```python
from build123d import *

# Parameters (mm, degrees)
SKETCH2_R           = 11.5
BOSS_EXTRUDE1_DEPTH = 1
SKETCH3_R           = 10
BOSS_EXTRUDE2_DEPTH = 4
SKETCH4_R           = 2.525
CUT_EXTRUDE1_DEPTH  = 17.984370982
SKETCH5_R           = 2
CUT_EXTRUDE2_DEPTH  = 0.3
CIRPATTERN1_COUNT   = 14
SKETCH7_R           = 10
SKETCH7_R_2         = 2.525
BOSS_EXTRUDE4_DEPTH = 1.5
BOSS_EXTRUDE3_DEPTH = 0.998
SKETCH8_R           = 1.1
CUT_EXTRUDE3_DEPTH  = 2.69
CUT_EXTRUDE4_DEPTH  = 1.7
CIRPATTERN2_COUNT   = 3
SKETCH11_R          = 11.5
BOSS_EXTRUDE5_DEPTH = 3
SKETCH12_R          = 1.65
CUT_EXTRUDE5_DEPTH  = 4
CUT_EXTRUDE6_DEPTH  = 2.8
CIRPATTERN3_COUNT   = 4
SKETCH16_R          = 4.5
CUT_EXTRUDE9_DEPTH  = 2
SKETCH17_R          = 3.5
CUT_EXTRUDE10_DEPTH = 18.866109191


with BuildPart() as part:
    # Sketch2 → Boss-Extrude1 (new body)
    with BuildSketch(Plane(origin=(0, 0, 0), x_dir=(1, 0, 0), z_dir=(0, 1, 0))):
        with Locations(Location((0, 0, 0), (0, 0, 270))):
            Circle(SKETCH2_R)
    extrude(amount=BOSS_EXTRUDE1_DEPTH)

    # Sketch3 → Boss-Extrude2 (add)
    with BuildSketch(Plane(origin=(0, 1, 0), x_dir=(1, 0, 0), z_dir=(0, 1, 0))):
        with Locations(Location((0, 0, 0), (0, 0, 270))):
            Circle(SKETCH3_R)
    extrude(amount=BOSS_EXTRUDE2_DEPTH)

    # Sketch4 → Cut-Extrude1 (cut, through all)
    with BuildSketch(Plane(origin=(0, 4.8958, 0), x_dir=(-1, 0, 0), z_dir=(0, -1, 0))):
        with Locations(Location((0, 7, 0), (0, 0, 90))):
            Circle(SKETCH4_R)
    cut_extrude1 = extrude(amount=-CUT_EXTRUDE1_DEPTH, mode=Mode.SUBTRACT)

    # Sketch5 → Cut-Extrude2 (cut)
    with BuildSketch(Plane(origin=(0, 4.8958, 0), x_dir=(1, 0, 0), z_dir=(0, 1, 0))):
        with Locations(Location((0, 7, 0), (0, 0, 270))):
            Circle(SKETCH5_R)
    cut_extrude2 = extrude(amount=-CUT_EXTRUDE2_DEPTH, mode=Mode.SUBTRACT)

    # CirPattern1: Cut-Extrude1, Cut-Extrude2 ×14 about axis, 11 skipped
    cirpattern1_axis = Axis((0, 5, 0), (0, -1, 0))
    add([cut_extrude1.rotate(cirpattern1_axis, i * 360 / CIRPATTERN1_COUNT) for i in range(1, CIRPATTERN1_COUNT) if i not in (1, 2, 3, 4, 6, 7, 8, 10, 11, 12, 13)], mode=Mode.SUBTRACT)
    add([cut_extrude2.rotate(cirpattern1_axis, i * 360 / CIRPATTERN1_COUNT) for i in range(1, CIRPATTERN1_COUNT) if i not in (1, 2, 3, 4, 6, 7, 8, 10, 11, 12, 13)], mode=Mode.SUBTRACT)

    # Sketch7 → Boss-Extrude4 (add)
    with BuildSketch(Plane(origin=(0, 4.8958, 0), x_dir=(1, 0, 0), z_dir=(0, 1, 0))):
        with Locations(Location((0, 0, 0), (0, 0, 270))):
            Circle(SKETCH7_R)
        with Locations(Location((5.472820377, -4.364428613, 0), (0, 0, 321.428571429))):
            Circle(SKETCH7_R_2, mode=Mode.SUBTRACT)
        with Locations(Location((-5.472820377, -4.364428613, 0), (0, 0, 90))):
            Circle(SKETCH7_R_2, mode=Mode.SUBTRACT)
        with Locations(Location((0, 7, 0), (0, 0, 90))):
            Circle(SKETCH7_R_2, mode=Mode.SUBTRACT)
    extrude(amount=BOSS_EXTRUDE4_DEPTH)

    # Sketch6 → Boss-Extrude3 (add)
    with BuildSketch(Plane(origin=(0, 6.3958, 0), x_dir=(1, 0, 0), z_dir=(0, 1, 0))):
        with BuildLine():
            ThreePointArc((-0.412808131, 9.491026786), (-2.524163057, 6.934993371), (-0.284039451, 4.491026786))
            ThreePointArc((-0.284039451, 4.491026786), (-4.054359906, 1.952476826), (-3.688321831, -2.578038415))
            ThreePointArc((-3.688321831, -2.578038415), (-6.995786073, -2.350427498), (-7.677765202, -5.594812017))
            ThreePointArc((-7.677765202, -5.594812017), (-8.559204245, 4.121895522), (-0.412808131, 9.491026786))
        make_face()
        with BuildLine():
            ThreePointArc((3.334130428, -3.022180386), (3.848206224, -6.297367788), (7.163001882, -6.240304803))
            ThreePointArc((7.163001882, -6.240304803), (0, -9.5), (-7.163001882, -6.240304803))
            ThreePointArc((-7.163001882, -6.240304803), (-3.848206224, -6.297367788), (-3.334130428, -3.022180386))
            ThreePointArc((-3.334130428, -3.022180386), (0, -4.5), (3.334130428, -3.022180386))
        make_face()
        with BuildLine():
            ThreePointArc((0.284039451, 4.491026786), (2.524163057, 6.934993371), (0.412808131, 9.491026786))
            ThreePointArc((0.412808131, 9.491026786), (8.559204245, 4.121895522), (7.677765202, -5.594812017))
            ThreePointArc((7.677765202, -5.594812017), (6.995786073, -2.350427498), (3.688321831, -2.578038415))
            ThreePointArc((3.688321831, -2.578038415), (4.054359906, 1.952476826), (0.284039451, 4.491026786))
        make_face()
    extrude(amount=BOSS_EXTRUDE3_DEPTH)

    # Sketch8 → Cut-Extrude3 (cut)
    with BuildSketch(Plane(origin=(0, 7.3938, 0), x_dir=(1, 0, 0), z_dir=(0, 1, 0))):
        with Locations(Location((0, -7, 0), (0, 0, 270))):
            Circle(SKETCH8_R)
    cut_extrude3 = extrude(amount=-CUT_EXTRUDE3_DEPTH, mode=Mode.SUBTRACT)

    # Sketch9 → Cut-Extrude4 (cut)
    with BuildSketch(Plane(origin=(0, 4.7038, 0), x_dir=(1, 0, 0), z_dir=(0, 1, 0))):
        Polygon((-1.975, -8.140266782), (-1.975, -11.329138317), (1.975, -11.329138317), (1.975, -8.140266782), (1.975, -5.859733218), (0, -4.719466437), (-1.975, -5.859733218), align=None)
    cut_extrude4 = extrude(amount=CUT_EXTRUDE4_DEPTH, mode=Mode.SUBTRACT)

    # CirPattern2: Cut-Extrude3, Cut-Extrude4 ×3 about axis
    cirpattern2_axis = Axis((0, 0, 0), (0, 1, 0))
    add([cut_extrude3.rotate(cirpattern2_axis, i * 360 / CIRPATTERN2_COUNT) for i in range(1, CIRPATTERN2_COUNT)], mode=Mode.SUBTRACT)
    add([cut_extrude4.rotate(cirpattern2_axis, i * 360 / CIRPATTERN2_COUNT) for i in range(1, CIRPATTERN2_COUNT)], mode=Mode.SUBTRACT)

    # Sketch11 → Boss-Extrude5 (add)
    with BuildSketch(Plane.XZ):
        with Locations(Location((0, 0, 0), (0, 0, 270))):
            Circle(SKETCH11_R)
    extrude(amount=BOSS_EXTRUDE5_DEPTH)

    # Sketch12 → Cut-Extrude5 (cut)
    with BuildSketch(Plane.XZ.offset(3)):
        with Locations(Location((0, 8, 0), (0, 0, 270))):
            Circle(SKETCH12_R)
    cut_extrude5 = extrude(amount=-CUT_EXTRUDE5_DEPTH, mode=Mode.SUBTRACT)

    # Sketch13 → Cut-Extrude6 (cut)
    with BuildSketch(Plane(origin=(0, 1, 0), x_dir=(1, 0, 0), z_dir=(0, 1, 0))):
        Polygon((-2.75, -9.58771324), (-2.75, -11.5), (2.75, -11.5), (2.75, -9.58771324), (2.75, -6.41228676), (0, -4.824573519), (-2.75, -6.41228676), align=None)
    cut_extrude6 = extrude(amount=-CUT_EXTRUDE6_DEPTH, mode=Mode.SUBTRACT)

    # CirPattern3: Cut-Extrude5, Cut-Extrude6 ×4 about axis
    cirpattern3_axis = Axis((0, 0, 0), (0, 1, 0))
    add([cut_extrude5.rotate(cirpattern3_axis, i * 360 / CIRPATTERN3_COUNT) for i in range(1, CIRPATTERN3_COUNT)], mode=Mode.SUBTRACT)
    add([cut_extrude6.rotate(cirpattern3_axis, i * 360 / CIRPATTERN3_COUNT) for i in range(1, CIRPATTERN3_COUNT)], mode=Mode.SUBTRACT)

    # Sketch16 → Cut-Extrude9 (cut)
    with BuildSketch(Plane(origin=(0, 6.3958, 0), x_dir=(1, 0, 0), z_dir=(0, 1, 0))):
        with Locations(Location((0, 0, 0), (0, 0, 93.618908364))):
            Circle(SKETCH16_R)
    extrude(amount=-CUT_EXTRUDE9_DEPTH, mode=Mode.SUBTRACT)

    # Sketch17 → Cut-Extrude10 (cut, through all)
    with BuildSketch(Plane(origin=(0, 4.3958, 0), x_dir=(1, 0, 0), z_dir=(0, 1, 0))):
        with Locations(Location((0, 0, 0), (0, 0, 270))):
            Circle(SKETCH17_R)
    extrude(amount=-CUT_EXTRUDE10_DEPTH, mode=Mode.SUBTRACT)


solid = part.part
```
Read the model definition and answer for the solid it produces. Units are mm, in the model's axes. A direction names the side the tool comes from. Round coordinates to 2 decimals unless told otherwise and drop trailing zeros. Write each loop counter-clockwise with the first axis right and the second up, starting at its lowest first coordinate (ties: lowest second). Pieces come first, ordered by that corner, then holes. Notation, with made-up numbers: (57, 82.5) - (100, 82.5) arc R31 cw to (100, 111.5) - close; hole circle Ø4 at (1, 20.25). An arc over 180 degrees is marked (long way). Use CSV: the item, a comma, the result in double quotes.
Q1. Find section A-A, the plane y = 6. Write down the section's boundary in (x, z) (3 decimals).
Values:
outline,"(-9.477, -3.191) - (-6.062, -1.219) - (-4.087, -2.36) - (-4.087, -4.64) - (-7.502, -6.612) arc R10 ccw to (7.502, -6.612) - (4.087, -4.64) - (4.087, -2.36) - (6.062, -1.219) - (9.477, -3.191) arc R10 ccw to (1.975, 9.803) - (1.975, 5.86) - (0, 4.719) - (-1.975, 5.86) - (-1.975, 9.803) arc R10 ccw to start; hole (-3.688, 2.578) arc R4.5 ccw to (-0.284, -4.491) arc R2.525 ccw (long way) to (0.284, -4.491) arc R4.5 ccw to (3.688, 2.578) arc R2.525 ccw (long way) to (3.334, 3.022) arc R4.5 ccw to (-3.334, 3.022) arc R2.525 ccw (long way) to start"
Q2. Find section D-D, the plane y = 3.5. Write down the section's boundary in (x, z), then the cut area to 3 significant figures.
Values:
outline,"circle Ø20 at (0, 0); hole circle Ø7 at (0, 0)"
area,"276 mm²"
Q3. Straight lines are drawn through the part: line 1 along Y through (x, z) = (4.5, -2.75); line 2 along X through (y, z) = (6.5, -6.25); line 3 along X through (y, z) = (6.5, -4). For each, find the intervals that lie inside material, in ascending order.
Values:
line 1,"y = -3 to 4.7, 6.4 to 7.39"
line 2,"x = -7.15 to -2.41, 2.41 to 7.15"
line 3,"x = -8.62 to -7.04, -5.08 to -2.06, 2.06 to 5.08, 7.04 to 8.62"
Q4. Find section B-B, the plane z = -5.5. Write down the section's boundary in (x, y), then the cut area to 3 significant figures.
Values:
outline,"(-10.1, -3) - (10.1, -3) - (10.1, 1) - (8.35, 1) - (8.35, 4.7) - (5.58, 4.7) - (5.58, 6.4) - (7.75, 6.4) - (7.75, 7.39) - (2.03, 7.39) - (2.03, 4.9) - (1.32, 4.9) - (1.32, 4.6) - (-1.32, 4.6) - (-1.32, 4.9) - (-2.03, 4.9) - (-2.03, 7.39) - (-7.75, 7.39) - (-7.75, 6.4) - (-5.58, 6.4) - (-5.58, 4.7) - (-8.35, 4.7) - (-8.35, 1) - (-10.1, 1) - close; hole (-1.17, -1.8) - (1.17, -1.8) - (1.17, 1) - (-1.17, 1) - close"
area,"159 mm²"
Q5. Find section C-C, the plane z = -8. Write down the section's boundary in (x, y), then the cut area to 3 significant figures.
Values:
outline,"(-8.26, -3) - (-1.65, -3) - (-1.65, -1.8) - (-2.75, -1.8) - (-2.75, 1) - (2.75, 1) - (2.75, -1.8) - (1.65, -1.8) - (1.65, -3) - (8.26, -3) - (8.26, 1) - (6, 1) - (6, 6.4) - (5.12, 6.4) - (5.12, 7.39) - (2.32, 7.39) - (2.32, 4.9) - (1.73, 4.9) - (1.73, 4.6) - (-1.73, 4.6) - (-1.73, 4.9) - (-2.32, 4.9) - (-2.32, 7.39) - (-5.12, 7.39) - (-5.12, 6.4) - (-6, 6.4) - (-6, 1) - (-8.26, 1) - close"
area,"109 mm²"
Q6. Determine the mould class of faces 4 (the cylindrical face through (1, 6.13, -4.68)), 5 (the flat face through (1, 6.404, 8)), 6 (the flat face through (-8, 1, 0)), 7 (the flat face through (5.63, -0.38, -1.394)) for opening direction X: +X half, -X half, draft (parallel to the pull), parting line (faces both ways), or undercut.
Values:
face 4,"undercut"
face 5,"undercut"
face 6,"draft"
face 7,"+X half"
Q7. A tool of negligible diameter and unlimited length cuts with its end or side. For faces 1 (the flat face through (-1.36, -0.38, 5.61)), 2 (the cylindrical face through (6.39, 6.91, -2.45)), 3 (the flat face through (7.3, 6.404, -3.7)), from which of +Z, -Z, +X, -X, +Y, -Y can it reach the whole face along a straight path? Write none if from no direction.
Values:
face 1,"+Z"
face 2,"+Y"
face 3,"none"
Q8. Each of these flat-tipped pins is pushed along its axis until it touches: pin 1 Ø6.5 at (x, z) = (0, 0) entering from +Y; pin 2 Ø0.5 at (y, z) = (5.5, 8) entering from +X; pin 3 Ø3 at (x, y) = (-3.5, 0.5) entering from -Z; pin 4 Ø1.2 at (x, z) = (5, 4.5) entering from +Y. Where does it stop, or does it pass through?
Values:
pin 1,"passes through"
pin 2,"stops at x = 6.32"
pin 3,"stops at z = -11.17"
pin 4,"stops at y = 4.6"
